The model under review builds one solid part; all positions refer to its coordinate system, in mm. A direction names the side the tool comes from. Round coordinates to 2 decimals unless told otherwise and drop trailing zeros. Loops run counter-clockwise (first coordinate to the right, second up) from the corner with the lowest first, then second, coordinate; pieces in that order, holes last. Notation, with made-up numbers: M 67.5,63 L 126.5,63 A35 cw 126.5,100 Z; hole C 15.25,-6.75 d8. An arc over 180 degrees is marked long. Return JSON: item names as keys, results as strings. Group by question number.
Q1. For faces 1 (the face through (-16, 3.6, -15.875)), 2 (the face through (-15.613, -6.905, -17.198)), 3 (the face through (-13.97, -11, -18)), list the 3-axis set-ups (+Z, -Z, +X, -X, +Y, -Y) from which the entire face can be reached by the end or side of a thin tool; tool diameter is ignored.
Q2. Consider section D-D (z = 10.5). State the section outline as (x, y) points (3 decimals).
Q3. Consider section B-B (z = 18.5). State the section outline as (x, y) points (3 decimals).
Q4. Clearance check with flat-ended pins moving along their axes: pin 1 Ø2 at (x, y) = (0, -4) entering from -Z; pin 2 Ø4 at (x, y) = (18.5, 4.5) entering from +Z (3 decimals); pin 3 Ø5 at (x, y) = (15.875, 6.35) entering from -Z (3 decimals); pin 4 Ø8 at (x, z) = (3.5, -4) entering from +Y. State where each tip first meets the part, or that it passes through.
Q5. Consider section A-A (y = 6.35). State the section outline as (x, z) points (3 decimals), and give its area (3 significant figures).
Q6. Draft analysis for pull direction X (two halves, no side actions). For faces 4 (the face through (13.97, -11, 18)), 5 (the face through (-16, 12.7, -19)), 6 (the face through (22.225, -5, -5)), state which applies: pulls with the +X half, pulls with the -X half, needs draft (parallel to the pull), parting line crosses it, or undercut.
Q7. Consider section C-C (y = -4). State the section outline as (x, z) points (3 decimals).
Q8. To check wall thickness, follow line 1 along X through (y, z) = (-9, -16.51) (3 decimals); line 2 along Z through (x, y) = (16.51, -6.25) (3 decimals). State the ranges of each line that lie inside material, in increasing order.
from build123d import *

# Parameters (mm, degrees)
F0_W     = 44.45
F0_H     = 44.45
F1_DEPTH = 12.7
F2_W     = 12.7
F2_H     = 6.35
F3_DEPTH = 12.7
F5_DEPTH = 2.54
F6_D     = 2.2606
F6_DEPTH = 11.43
F6_TIP   = 0.6791527577
F9_DEPTH = 12.701
F10_D    = 4.4958


# Not quite as in the source:
# - a pattern or mirror of a feature is missing from the dataset's text; its kind, count and spacing are read off the source's solid


with BuildPart() as f1:
    # F0 (on Front) → F1 (new body)
    with BuildSketch(Plane.XZ):
        Rectangle(F0_W, F0_H)
    extrude(amount=F1_DEPTH)

    # F2 (on face) → F3 (join)
    with BuildSketch(Plane(origin=(-22.225, 0, 0), x_dir=(0, -1, 0), z_dir=(-1, 0, 0))):
        with Locations((-6.35, -19.05)):
            Rectangle(F2_W, F2_H)
    f3 = extrude(amount=-F3_DEPTH)

    # F3_copies: F3 across plane
    add(f3.mirror(Plane(origin=(0, 0, 0), x_dir=(0, 0, 1), z_dir=(1, 0, 0))))

    # F4 (on face) → F5 (cut)
    with BuildSketch(Plane.XZ.offset(12.7)):
        Polygon((-13.97, 13.97), (-22.225, 13.97), (-22.225, 0), (-22.225, -13.97), (-13.97, -13.97), (-13.97, -22.225), (0, -22.225), (13.97, -22.225), (13.97, -13.97), (22.225, -13.97), (22.225, 0), (22.225, 13.97), (13.97, 13.97), (13.97, 22.225), (0, 22.225), (-13.97, 22.225), align=None)
    extrude(amount=-F5_DEPTH, mode=Mode.SUBTRACT)

    # F6
    with Locations(Plane.XZ.offset(12.7)):
        with Locations((-16.51, 16.51), (16.51, 16.51), (16.51, -16.51), (-16.51, -16.51)):
            Hole(F6_D / 2, depth=F6_DEPTH)
            with Locations((0, 0, -(F6_DEPTH + F6_TIP / 2))):  # 118° drill point
                Cone(0, F6_D / 2, F6_TIP, mode=Mode.SUBTRACT)

    # F8 (on face) → F9 (cut, through all)
    with BuildSketch(Plane(origin=(0, 0, 0), x_dir=(-1, 0, 0), z_dir=(0, 1, 0))):
        with BuildLine():
            Line((-9.525, 3.175), (-9.525, -22.225))
            Line((-9.525, -22.225), (9.525, -22.225))
            Line((9.525, -22.225), (9.525, 3.175))
            ThreePointArc((9.525, 3.175), (0, 12.7), (-9.525, 3.175))
        make_face()
    extrude(amount=-F9_DEPTH, mode=Mode.SUBTRACT)

    # F10 (through all)
    with Locations(Plane(origin=(0, 0, -22.225), x_dir=(1, 0, 0), z_dir=(0, 0, -1))):
        with Locations((15.875, -6.35)):
            f10 = Hole(F10_D / 2)

    # F10_copies: F10 across plane
    add(f10.mirror(Plane(origin=(0, 0, 0), x_dir=(0, 0, -1), z_dir=(-1, 0, 0))), mode=Mode.SUBTRACT)


solid = f1.part
Values:
{
 "1": {"face 1": "+Z, +X, -X, +Y", "face 2": "-Y", "face 3": "+Z, -Z, -Y"},
 "2": {"outline": "M -22.225,-10.16 L -6.089,-10.16 L -6.089,0 L -22.225,0 Z; M 6.089,-10.16 L 22.225,-10.16 L 22.225,0 L 6.089,0 Z"},
 "3": {"outline": "M -22.225,-12.7 L -13.97,-12.7 L -13.97,-10.16 L 13.97,-10.16 L 13.97,-12.7 L 22.225,-12.7 L 22.225,0 L -22.225,0 Z"},
 "4": {"pin 1": "stops at z = 12.65", "pin 2": "stops at z = -15.875", "pin 3": "stops at z = -22.225", "pin 4": "passes through"},
 "5": {"outline": "M -22.225,-22.225 L -18.123,-22.225 L -18.123,-15.875 L -22.225,-15.875 Z; M -13.627,-22.225 L -9.525,-22.225 L -9.525,-15.875 L -13.627,-15.875 Z; M 9.525,-22.225 L 13.627,-22.225 L 13.627,-15.875 L 9.525,-15.875 Z; M 18.123,-22.225 L 22.225,-22.225 L 22.225,-15.875 L 18.123,-15.875 Z", "area": "104 mm2"},
 "6": {"face 4": "undercut", "face 5": "needs draft", "face 6": "pulls with the +X half"},
 "7": {"outline": "M -22.225,-22.225 L -9.525,-22.225 L -9.525,3.175 A9.525 cw 9.525,3.175 L 9.525,-22.225 L 22.225,-22.225 L 22.225,22.225 L -22.225,22.225 Z; hole C -16.51,-16.51 d2.261; hole C -16.51,16.51 d2.261; hole C 16.51,-16.51 d2.261; hole C 16.51,16.51 d2.261"},
 "8": {"line 1": "x = -22.225 to -17.64, -15.38 to -9.525, 9.525 to 15.38, 17.64 to 22.225", "line 2": "z = -22.225 to -17.64, -15.38 to 15.38, 17.64 to 22.225"}
}
